CAD build for the part. Positions are in the model's coordinates, mm. Give positions to 0.01 mm unless a question says otherwise; leave off trailing zeros. Write each loop counter-clockwise with the first axis right and the second up, starting at its lowest first coordinate (ties: lowest second). Pieces come first, ordered by that corner, then holes. Notation, with made-up numbers: M 37.5,40 L 79.5,40 A7 cw 79.5,47 Z; hole C -13,-20.75 d11. An arc over 180 degrees is marked long. One line per question, with ' | ' between items. Start each with the question number.
1. Cut at B-B, the plane y = 29. Write the cut outline in (x, z).
2. Cut at C-C, the plane z = 41. Write the cut outline in (x, y), then the cut area to 3 significant figures.
3. Wall check: L1, parallel to Z at x = 63, y = 4; L2, parallel to X at y = 7, z = 0; L3, parallel to X at y = 28, z = 0. Give the ranges that are in metal, low to high.
4. Cut at D-D, the plane x = -155. Write the cut outline in (y, z).
5. Flat gauge pins, fed straight in: pin 1 (2 mm diameter, centred on x = 14.5, z = 94.5, fed in from +Y); pin 2 (3 mm diameter, centred on x = -9, y = 31.5, fed in from +Z); pin 3 (12 mm diameter, centred on x = -69.5, z = 53, fed in from -Y). Where does each tip first touch, or does it go through?
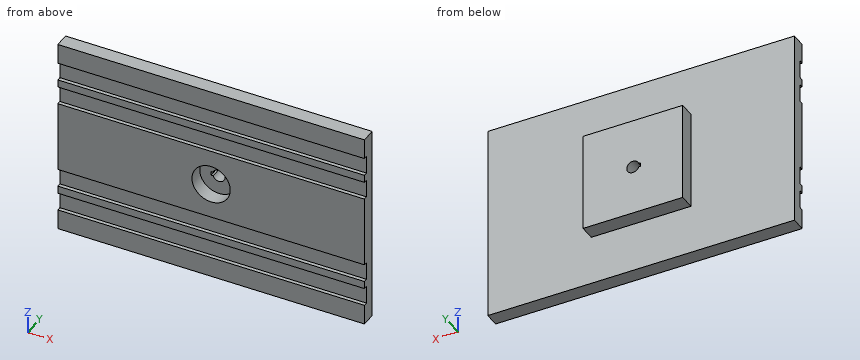
```python
from build123d import *

# Parameters (mm, degrees)
SKETCH1_W           = 400
SKETCH1_H           = 260
BOSS_EXTRUDE1_DEPTH = 19
SKETCH2_W           = 400
SKETCH2_H           = 23.6
CUT_EXTRUDE1_DEPTH  = 5
SKETCH4_W           = 130
SKETCH4_H           = 130
BOSS_EXTRUDE4_DEPTH = 20
SKETCH5_R           = 8
CUT_EXTRUDE2_DEPTH  = 242.704364876
SKETCH6_W           = 2.5
SKETCH6_H           = 5
CUT_EXTRUDE4_DEPTH  = 242.704364876
SKETCH7_R           = 25
CUT_EXTRUDE5_DEPTH  = 19


with BuildPart() as part:
    # Sketch1 → Boss-Extrude1 (new body)
    with BuildSketch(Plane(origin=(0, 0, 0), x_dir=(1, 0, 0), z_dir=(0, 1, 0))):
        Rectangle(SKETCH1_W, SKETCH1_H)
    extrude(amount=BOSS_EXTRUDE1_DEPTH)

    # Sketch2 → Cut-Extrude1 (cut)
    with BuildSketch(Plane.XZ):
        with Locations((0, 91.8)):
            Rectangle(SKETCH2_W, SKETCH2_H)
        with Locations((0, 58.2)):
            Rectangle(SKETCH2_W, SKETCH2_H)
        with Locations((0, -58.2)):
            Rectangle(SKETCH2_W, SKETCH2_H)
        with Locations((0, -91.8)):
            Rectangle(SKETCH2_W, SKETCH2_H)
    extrude(amount=-CUT_EXTRUDE1_DEPTH, mode=Mode.SUBTRACT)

    # Sketch4 → Boss-Extrude4 (add)
    with BuildSketch(Plane(origin=(0, 19, 0), x_dir=(1, 0, 0), z_dir=(0, 1, 0))):
        Rectangle(SKETCH4_W, SKETCH4_H)
    extrude(amount=BOSS_EXTRUDE4_DEPTH)

    # Sketch5 → Cut-Extrude2 (cut, through all)
    with BuildSketch(Plane(origin=(0, 39, 0), x_dir=(1, 0, 0), z_dir=(0, 1, 0))):
        with Locations(Location((0, 0, 0), (0, 0, 270))):
            Circle(SKETCH5_R)
    extrude(amount=-CUT_EXTRUDE2_DEPTH, mode=Mode.SUBTRACT)

    # Sketch6 → Cut-Extrude4 (cut, through all)
    with BuildSketch(Plane(origin=(0, 39, 0), x_dir=(1, 0, 0), z_dir=(0, 1, 0))):
        with Locations((-8.849342077, 0)):
            Rectangle(SKETCH6_W, SKETCH6_H)
    extrude(amount=-CUT_EXTRUDE4_DEPTH, mode=Mode.SUBTRACT)

    # Sketch7 → Cut-Extrude5 (cut)
    with BuildSketch(Plane.XZ):
        with Locations(Location((0, 0, 0), (0, 0, 270))):
            Circle(SKETCH7_R)
    extrude(amount=-CUT_EXTRUDE5_DEPTH, mode=Mode.SUBTRACT)


solid = part.part
```
Here are the results:
1) outline: M -65,-65 L 65,-65 L 65,65 L -65,65 Z; hole M -10.1,-2.5 L -7.6,-2.5 A8 ccw long -7.6,2.5 L -10.1,2.5 Z
2) outline: M -200,0 L 200,0 L 200,19 L 65,19 L 65,39 L -65,39 L -65,19 L -200,19 Z | area: 10,200 mm^2
3) L1: -130 to -103.6, -80 to -70, -46.4 to 46.4, 70 to 80, 103.6 to 130 | L2: -200 to -25, 25 to 200 | L3: -65 to -10.1, 8 to 65
4) outline: M 0,-130 L 19,-130 L 19,130 L 0,130 L 0,103.6 L 5,103.6 L 5,80 L 0,80 L 0,70 L 5,70 L 5,46.4 L 0,46.4 L 0,-46.4 L 5,-46.4 L 5,-70 L 0,-70 L 0,-80 L 5,-80 L 5,-103.6 L 0,-103.6 Z
5) pin 1: y = 19 | pin 2: z = 65 | pin 3: y = 5
